Job drawing, mm, ordinate dimensions from the low corner. One solid piece. A direction names the side the tool comes from. Round coordinates to 2 decimals unless told otherwise and drop trailing zeros. Order: outer loops, then holes, each group sorted by start corner. A loop starts at its lowest first (then second) coordinate and runs counter-clockwise, first axis right, second up. Notation, with made-up numbers: (-34.75, 20.5) -> (4.25, 20.5) arc R15 ccw to (4.25, 25.5) -> close; hole circle Ø11 at (-6.75, 34). An arc over 180 degrees is marked (long way). Write item = value, one per line.
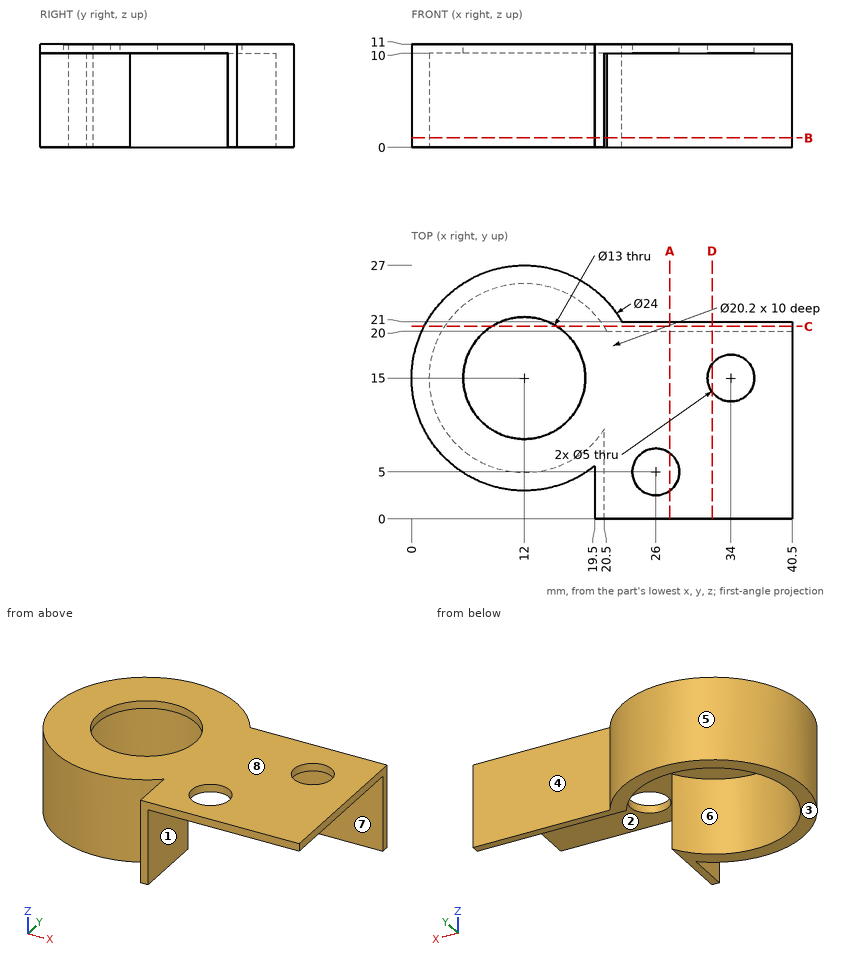
Q1. Cut at D-D, the plane x = 32. List the corners of the cut face in (y, z).
Check values:
outline = (0, 10) -> (13.5, 10) -> (13.5, 11) -> (0, 11) -> close; (16.5, 10) -> (20, 10) -> (20, 0) -> (21, 0) -> (21, 11) -> (16.5, 11) -> close
Q2. Mould opens along X. For the marked faces 1, 2 and 3 say: released by +X, released by -X, zero draft, split by the parting line, or undercut.
Check values:
face_1 = released by +X
face_2 = undercut
face_3 = zero draft
Q3. Cut at B-B, the plane z = 1. List the corners of the cut face in (x, y), and give its area (3 significant figures).
Check values:
outline = (19.5, 0) -> (20.5, 0) -> (20.5, 9.54) arc R10.1 cw (long way) to (20.78, 20) -> (40.5, 20) -> (40.5, 21) -> (22.39, 21) arc R12 ccw (long way) to (19.5, 5.63) -> close
area = 131 mm²
Q4. Which spindle directions (+Z, -Z, +X, -X, +Y, -Y) get a long thin tool onto all of the face, cutting with end or side? Do the marked faces 4, 5, 6, 7 and 8. Say none if no direction does.
Check values:
face_4 = +Z, -Z, +X, +Y
face_5 = +Z, -Z
face_6 = -Z
face_7 = -Z, +X, -Y
face_8 = +Z, +X, -X, +Y, -Y
Q5. Cut at C-C, the plane y = 20.5. List the corners of the cut face in (x, z), and give its area (3 significant figures).
Check values:
outline = (1.33, 0) -> (3.53, 0) -> (3.53, 10) -> (8.54, 10) -> (8.54, 11) -> (1.33, 11) -> close; (15.46, 10) -> (20.47, 10) -> (20.47, 0) -> (40.5, 0) -> (40.5, 11) -> (15.46, 11) -> close
area = 254 mm²
Q6. Probe probe 1 along Y at (x, z) = (34, 10.65); probe 2 along Y at (x, z) = (28, 4.5); probe 3 along Z at (x, y) = (30.5, 10.25). List the from-to ranges inside material, lowest first.
Check values:
probe_1 = 0 to 12.5, 17.5 to 21
probe_2 = 20 to 21
probe_3 = 10 to 11
Q7. Cut at A-A, the plane x = 27.5. List the corners of the cut face in (y, z), and give its area (3 significant figures).
Check values:
outline = (0, 10) -> (3, 10) -> (3, 11) -> (0, 11) -> close; (7, 10) -> (20, 10) -> (20, 0) -> (21, 0) -> (21, 11) -> (7, 11) -> close
area = 27.0 mm²
Q8. Flat gauge pins, fed straight in: pin 1 (8 mm diameter, centred on x = 26, y = 14.5, fed in from -Z); pin 2 (5 mm diameter, centred on y = 6.5, z = 10, fed in from -X); pin 3 (4.5 mm diameter, centred on y = 2, z = 8, fed in from -X); pin 4 (4.5 mm diameter, centred on x = 26, y = 5, fed in from -Z). Where does each tip first touch, or does it go through?
Check values:
pin_1 = 10
pin_2 = 1.61
pin_3 = 6.67
pin_4 = through
